Input: part model. Units: mm. Frame: model coordinates. A direction names the side the tool comes from. Round coordinates to 2 decimals unless told otherwise and drop trailing zeros. Loops run counter-clockwise (first coordinate to the right, second up) from the corner with the lowest first, then second, coordinate; pieces in that order, holes last. Notation, with made-up numbers: M 68.5,17.25 L 112.5,17.25 A18 cw 112.5,41.25 Z; hole C 38,-9.75 d10. An arc over 180 degrees is marked long. Use one line per item in the form item = value. Start each with the question number.
Q1. Mould query, pull axis X, two halves, no side actions, for faces 1 (the flat face through (0, 0, 2)), 2 (the cylindrical face through (1.97, 24.42, -13.72)), 3 (the flat face through (-7, 9, 2)). Classes: pulls with the +X half, pulls with the -X half, needs draft (parallel to the pull), parting line crosses it, or undercut.
Q2. Access query for faces 4 (the flat face through (-38, -2, -14)), 5 (the flat face through (22, -2, -14)), 6 (the flat face through (-26, 5, 0)), 7 (the cylindrical face through (2.192, -4.214, -27.986)). Directions: +Z, -Z, +X, -X, +Y, -Y. A direction counts if a zero-diameter tool reaches every point of the face in a straight line with its end or side. Return the directions, or none.
Q3. Section query B-B, the plane y = 15. Output: boundary loops of the cut face in (x, z).
Q4. Section query C-C, the plane x = -14.5. Output: boundary loops of the cut face in (y, z), and give its area (3 significant figures).
Q5. First-contact query: P1, Ø9, axis at x = -37.5, z = -8, coming from the +Y side; P2, Ø4, axis at x = 15.5, z = -12.5, coming from the -Y side; P3, Ø5.5, axis at x = 0, y = 0, coming from the -Z side; P4, Ø3.5, axis at x = -49.42, z = -5.5, coming from the -Y side. Flat tips, straight axial feed; report the tip coordinate or a pass-through.
Q6. Ray query, line 1 along X through (y, z) = (-0.5, -13.5); line 2 along Z through (x, y) = (3, 20); line 3 along X through (y, z) = (2, -13). Return the intervals inside material, ascending.
Autodesk Inventor part; units mm, degrees
ref_plane "Work Plane2" through (0, 0, -13.5) normal (0, 0, 1) x (1, 0, 0)
ref_plane "YZ Plane" through (0, 0, 0) normal (1, 0, 0) x (0, 1, 0)
ref_plane "XZ Plane" through (0, 0, 0) normal (0, 1, 0) x (-1, 0, 0)
sketch "Sketch1" plane through (0, 0, 0) normal (0, 0, 1) x (1, 0, 0)
  circle A0 centre (0, 0) radius 4.75
  circle A1 centre (0, 0) radius 17.5 construction
  arc A2 (20.4022, -2) -> (-20.4022, -2) centre (0, 0) ccw
  arc A3 (-20.4022, -2) -> (20.4022, -2) centre (0, 33.0909) ccw
  arc A4 (-20.4022, -2) -> (20.4022, -2) centre (0, 0) ccw construction
  arc A5 (24.4182, -2) -> (-24.4182, -2) centre (0, 0) ccw
  line L0 (-20.4022, -2) -> (-24.4182, -2)
  line L1 (20.4022, -2) -> (24.4182, -2)
  arc A6 (-24.4182, -2) -> (24.4182, -2) centre (0, 0) ccw construction
  dimension "d0" = 9.5
  dimension "d1" = 35
  dimension "d2" = 41
  dimension "d3" = 10
  dimension "d4" = 2
  dimension "d5" = 49
extrude "Extrusion1" add sketch "Sketch1" along normal blind 2
extrude "Extrusion2" add sketch "Sketch1" against normal blind 13.5 contours A2 L0 A5 L1
mirror "Mirror1" about plane through (0, 12.5652, -13.5) normal (0, 0, -1) of "Extrusion1", "Extrusion2"
sketch "Sketch2" plane through (0, 0, -29) normal (0, 0, -1) x (-1, 0, 0)
  circle A0 centre (0, 0) radius 7.45
  circle A1 centre (7.45, 0) radius 1
  circle A2 centre (-7.45, 0) radius 1
  point P0 (0, 7.45)
  dimension "d10" = 14.9
  dimension "d11" = 2
  dimension "d14" = 360
  dimension "d16" = 90
extrude "Extrusion3" cut sketch "Sketch2" against normal up to surface (2 mm away) contours A0 A1 | A0 A1 | A2 A0 | A0 A2
sketch "Sketch3" plane through (0, 0, 2) normal (0, 0, 1) x (1, 0, 0)
  circle A0 centre (0, 0) radius 7.5
  dimension "d19" = 15
extrude "Extrusion4" add sketch "Sketch3" along normal blind 1
fillet "Fillet1" radius 1 1 edges at (-7.5, 0, 3)
sketch "Sketch7" plane through (-24.4182, -2, 2) normal (0, -1, 0) x (1, 0, 0)
  line L0 (4.016, -2) -> (4.016, 0)
  line L1 (0, 0) -> (4.016, 0)
  line L2 (0, -31) -> (0, 0)
  line L3 (0, -31) -> (4.016, -31)
  line L4 (4.016, -29) -> (4.016, -31)
  line L5 (4.016, -2) -> (4.016, -29)
  line L6 (44.8204, -31) -> (4.016, -31)
  line L7 (4.016, -31) -> (-30, -31)
  line L8 (-30, -31) -> (-30, 0)
  line L9 (-30, 0) -> (4.016, 0)
  line L10 (4.016, 0) -> (4.016, -31)
  point P0 (24.4182, -2)
  dimension "d36" = 30
extrude "Extrusion8" add sketch "Sketch7" against normal blind 5
sketch "Sketch8" plane through (0, 33.0909, -29) normal (0, 0, -1) x (-1, 0, 0)
  arc A0 (24.3156, -30.0909) -> (-24.4182, -35.0909) centre (0, -33.0909) ccw
  line L0 (-20.4022, -35.0909) -> (-24.4182, -35.0909)
  arc A1 (-20.4022, -35.0909) -> (20.4022, -35.0909) centre (0, 0) ccw
  line L1 (54.4182, -35.0909) -> (20.4022, -35.0909)
  line L2 (54.4182, -35.0909) -> (54.4182, -30.0909)
  line L3 (24.3156, -30.0909) -> (54.4182, -30.0909)
  circle A2 centre (-7.45, -33.0909) radius 1
  circle A3 centre (7.45, -33.0909) radius 1
  circle A4 centre (0, -33.0909) radius 4.75
  arc A5 (24.3156, -30.0909) -> (-24.4182, -35.0909) centre (0, -33.0909) ccw
  line L4 (21.8918, -22.0909) -> (32.3156, -30.0909)
  line L5 (54.4182, -30.0909) -> (24.3156, -30.0909)
  dimension "d39" = 8
  dimension "d40" = 8
extrude "Extrusion9" add sketch "Sketch8" against normal blind 2 contours A0 L4 L3
ref_plane "Work Plane2" through (0, 0, -13.5) normal (0, 0, 1) x (1, 0, 0)
mirror "Mirror4" about plane through (0, 0, -13.5) normal (0, 0, 1) of "Extrusion9"
sketch "Sketch9" plane through (-24.4182, 3, 2) normal (0, 1, 0) x (1, 0, 0)
  line L0 (-7.8974, 0) -> (-7.8974, 2)
  line L1 (-7.8974, 2) -> (0.1026, 2)
  line L2 (0.1026, 29) -> (0.1026, 2)
  line L3 (0.1026, 29) -> (-7.8974, 29)
  line L4 (-7.8974, 29) -> (-7.8974, 31)
  line L5 (-7.8974, 31) -> (-30, 31)
  line L6 (-30, 31) -> (-30, 0)
  line L7 (-30, 0) -> (-7.8974, 0)
  point P0 (24.4182, 2)
  point P1 (-25, 7.5)
  point P2 (-25, 15.5)
  point P3 (-25, 23.5)
  point P4 (-9, 7.5)
  point P5 (-9, 15.5)
  point P6 (-9, 23.5)
  dimension "d45" = 8
  dimension "d48" = 16
  dimension "d51" = 31
  dimension "d52" = 7.5
  dimension "d53" = 5
hole "Hole1" at (-49.4182, 3, -5.5) at (-49.4182, 3, -13.5) at (-49.4182, 3, -21.5) at (-33.4182, 3, -5.5) at (-33.4182, 3, -13.5) at (-33.4182, 3, -21.5) direction (0, -1, 0) diameter 3.7 end through all
properties part number "Omni Encoder-trackers"
Results found:
q1.face_1 = undercut
q1.face_2 = parting line crosses it
q1.face_3 = needs draft
q2.face_4 = +Z, -Z, -X, -Y
q2.face_5 = +Z, -Z, +X, -Y
q2.face_6 = -X, +Y
q2.face_7 = -Z
q3.outline = M -19.37,-29 L 19.37,-29 L 19.37,2 L -19.37,2 Z; hole M -13.97,-27 L 13.97,-27 L 13.97,0 L -13.97,0 Z
q4.outline = M -4.82,-29 L 19.75,-29 L 19.75,2 L -4.82,2 L -4.82,0 L 14.49,0 L 14.49,-27 L -4.82,-27 Z
q4.area = 240 mm²
q5.P1 = 3
q5.P2 = 10.68
q5.P3 = 2
q5.P4 = through
q6.line_1 = -54.42 to -51.27, -47.57 to -35.27, -31.57 to -20.4, 20.49 to 24.49
q6.line_2 = -29 to -27, 0 to 2
q6.line_3 = -54.42 to -51.2, -47.64 to -35.2, -31.64 to -20.4, 20.4 to 24.42
